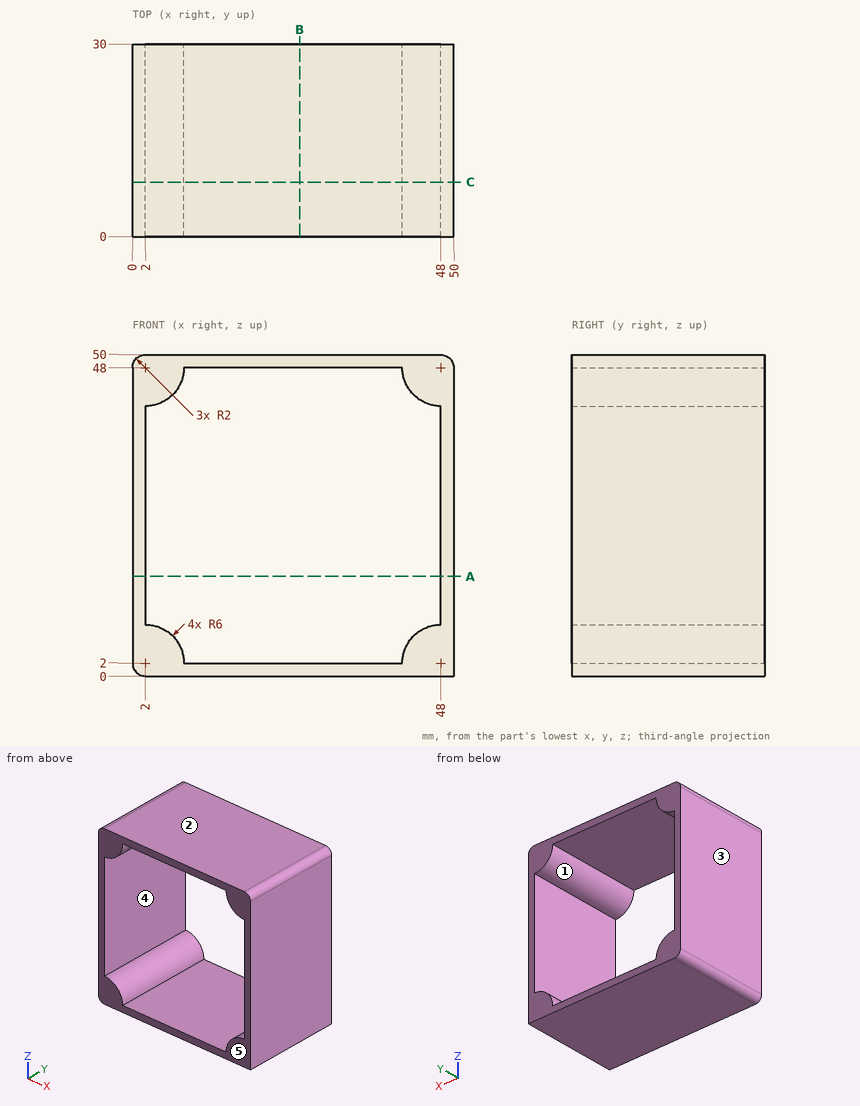
Study the drawing (mm; zero at the part's minimum x, y, z) and answer. A direction names the side the tool comes from. Round coordinates to 2 decimals unless told otherwise and drop trailing zeros. Write each loop counter-clockwise with the first axis right and the second up, starting at its lowest first coordinate (ties: lowest second). Pieces come first, ordered by that corner, then holes.
Q1. Find section B-B on x = 26. Determine the outline of the cut face in (y, z).
Values:
outline: (0, 0) - (30, 0) - (30, 2) - (0, 2) - close; (0, 48) - (30, 48) - (30, 50) - (0, 50) - close
Q2. Find section A-A on z = 15.5. Determine the outline of the cut face in (x, y).
Values:
outline: (0, 0) - (2, 0) - (2, 30) - (0, 30) - close; (48, 0) - (50, 0) - (50, 30) - (48, 30) - close
Q3. A flat-ended cylindrical pin translates along its axis: P1, Ø15, axis at y = 22, z = 27, coming from the -X side. Find the tip coordinate at first contact, or state that the pin passes through.
Values:
P1: stops at x = 0
Q4. The mould has two halves that part along X. Classify the marked faces 1, 2 and 3: released by +X, released by -X, zero draft, split by the parting line, or undercut.
Values:
face 1: undercut
face 2: zero draft
face 3: released by -X
Q5. Find section C-C on y = 8.5. Determine the outline of the cut face in (x, z), and give its area (3 significant figures).
Values:
outline: (0, 2) arc R2 ccw to (2, 0) - (50, 0) - (50, 48) arc R2 ccw to (48, 50) - (2, 50) arc R2 ccw to (0, 48) - close; hole (2, 8) arc R6 cw to (8, 2) - (42, 2) arc R6 cw to (48, 8) - (48, 42) arc R6 cw to (42, 48) - (8, 48) arc R6 cw to (2, 42) - close
area: 495 mm2
Q6. A tool of negligible diameter and unlimited length cuts with its end or side. For the marked faces 4 and 5, from which of +Z, -Z, +X, -X, +Y, -Y can it reach the whole face along a straight path? Write none if from no direction.
Values:
face 4: +Y, -Y
face 5: +Z, -Z, +X, -X, -Y
Q7. Straight lines are drawn through the part: line 1 (Z direction, x = 41, y = 24.75); line 2 (X direction, y = 2, z = 46). For each, find the intervals that lie inside material, in ascending order.
Values:
line 1: z = 0 to 2, 48 to 50
line 2: x = 0 to 7.66, 42.34 to 50
